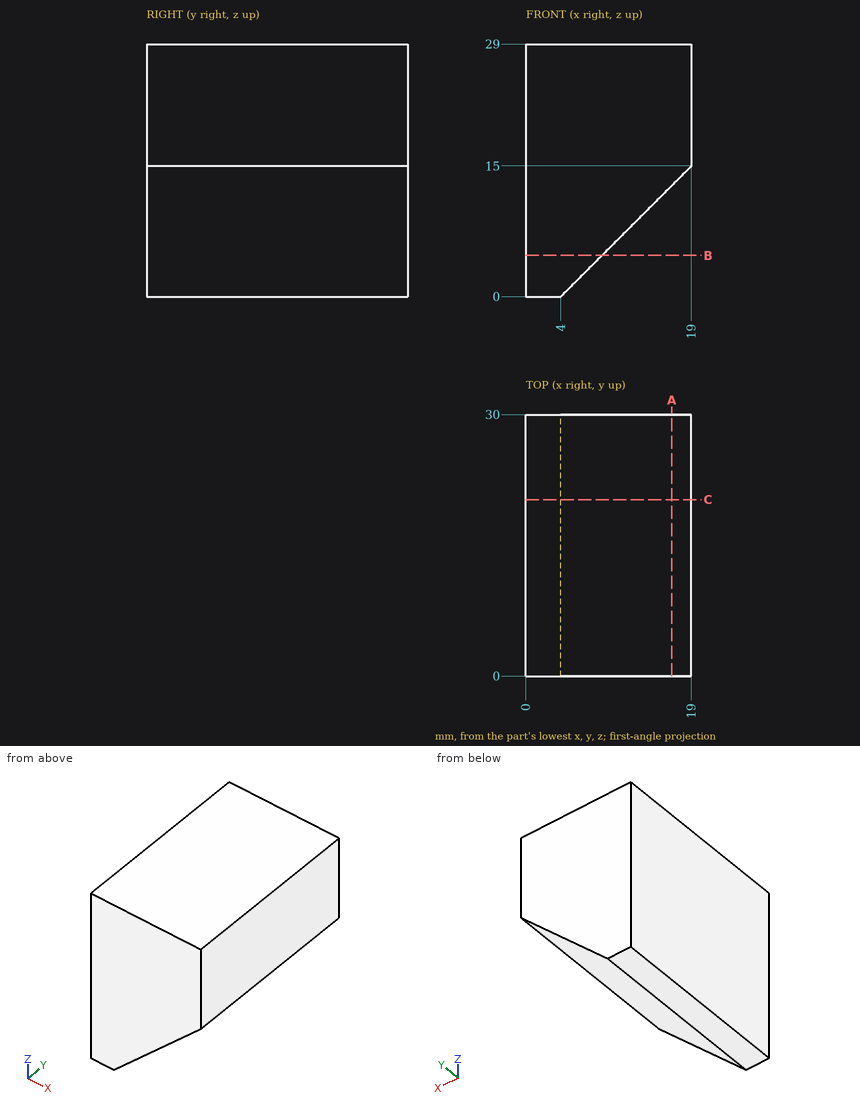
Study the drawing (mm; zero at the part's minimum x, y, z) and answer. Give positions to 0.01 mm unless a question says otherwise; leave off trailing zeros. Order: outer loops, then holes, each group sorted by start corner. A loop starts at its lowest first (then second) coordinate and runs counter-clockwise, first axis right, second up. Notation, with made-up numbers: (9, -29.75) - (49, -29.75) arc R23 cw to (49, -0.75) - close; hole circle Ø1 at (49.5, 58.25). An arc over 180 degrees is marked (long way). Use one line per item in the form item = value. Start each with the question number.
(1) A cutting plane is placed at C-C, the plane y = 20.25. Write down the section's boundary in (x, z), then the cut area to 4 significant figures.
(2) Consider line 1 (Z direction, x = 18.25, y = 20); line 2 (X direction, y = 17.5, z = 10.75); line 3 (X direction, y = 19.75, z = 12.75). Determine where each line is inside the solid, lowest interval first. Write a range as from..to.
(3) A cutting plane is placed at B-B, the plane z = 4.75. Write down the section's boundary in (x, y).
(4) A cutting plane is placed at A-A, the plane x = 16.75. Write down the section's boundary in (y, z).
Ans:
q1.outline = (0, 0) - (4, 0) - (19, 15) - (19, 29) - (0, 29) - close
q1.area = 438.5 mm^2
q2.line_1 = 14.25..29
q2.line_2 = 0..14.75
q2.line_3 = 0..16.75
q3.outline = (0, 0) - (8.75, 0) - (8.75, 30) - (0, 30) - close
q4.outline = (0, 12.75) - (30, 12.75) - (30, 29) - (0, 29) - close
